The listing builds one solid part. Answer for the finished solid, in the listing's coordinates (mm). A direction names the side the tool comes from. Give positions to 0.01 mm unless a question says otherwise; leave off trailing zeros. Loops run counter-clockwise (first coordinate to the right, second up) from the corner with the lowest first, then second, coordinate; pieces in that order, holes last.
Item 1: Section D-D, the plane x = 0.5 is taken. Give the vertices of the cut face in (y, z), and give its area (3 significant figures).
Item 2: Consider line 1 along X through (y, z) = (-8.25, -46.5); line 2 along Y through (x, z) = (10, -69); line 3 along X through (y, z) = (4.25, -75.5). Determine where each line is inside the solid, lowest interval first.
Item 3: A tool of negligible diameter and unlimited length cuts with its end or side. For faces 5 (the face through (20, -6, -49)), 6 (the face through (13.9, 0, -51)), 7 (the face through (-14, -8.2, -51)), 8 (the face through (-16, -10, -49)), 9 (the face through (10, 3.9, -51)), from which of +Z, -Z, +X, -X, +Y, -Y can it reach the whole face along a straight path? Write none if from no direction.
Item 4: Section C-C, the plane z = -82.5 is taken. Give the number of separate pieces and of enclosed holes in the cut face, and give its area (3 significant figures).
Item 5: Section A-A, the plane x = -10 is taken. Give the vertices of the cut face in (y, z), and give its area (3 significant figures).
Item 6: Section B-B, the plane y = 0 is taken. Give the vertices of the cut face in (x, z), and give its area (3 significant figures).
Item 7: Each of these flat-tipped pins is pushed along its axis until it touches: pin 1 Ø4.5 at (y, z) = (0.5, -52) entering from +X; pin 2 Ø3 at (y, z) = (0.5, -35.5) entering from -X; pin 3 Ø1.2 at (x, z) = (10, -46.5) entering from +Y. Where does it stop, or does it pass through?
Item 8: The mould has two halves that part along Y. Classify faces 1 (the face through (0, -10, -49)), 2 (the face through (-5, 5, 0)), 3 (the face through (-4.49, -4.45, -50.7)), 4 (the face through (5.52, -5.54, -50.7)): pulls with the +Y half, pulls with the -Y half, needs draft (parallel to the pull), parting line crosses it, or undercut.
from build123d import *

# Parameters (mm, degrees)
SKETCH2_W               = 40
SKETCH2_H               = 20
BOSS_EXTRUDE1_DEPTH     = 100
CUT_EXTRUDE1_DEPTH      = 103.46950766
CUT_EXTRUDE1_DEPTH_BACK = 103.46950766
SKETCH3_R               = 2.5
FILLET1_R               = 1.5


with BuildPart() as part:
    # Sketch2 → Boss-Extrude1 (new body)
    with BuildSketch(Plane.XY):
        Rectangle(SKETCH2_W, SKETCH2_H)
    extrude(amount=-BOSS_EXTRUDE1_DEPTH)

    # Sketch3 → Cut-Extrude1 (cut, two sides: drawn at the far end of the back side and taken through both)
    with BuildSketch(Plane.XY.offset(-CUT_EXTRUDE1_DEPTH_BACK)):
        with Locations((-10, 0)):
            Circle(SKETCH3_R)
        with Locations(Location((10, 0, 0), (0, 0, 180))):
            Circle(SKETCH3_R)
        with BuildLine():
            Line((-13.6, 10), (-6.4, 10))
            Line((-6.4, 10), (-6.4, 9.7))
            ThreePointArc((-6.4, 9.7), (-6.458578644, 9.558578644), (-6.6, 9.5))
            Line((-6.6, 9.5), (-6.9, 9.5))
            Line((-6.9, 9.5), (-6.9, 8.2))
            Line((-6.9, 8.2), (-4.5, 8.2))
            Line((-4.5, 8.2), (-4.5, 6.560660172))
            Line((-4.5, 6.560660172), (-6.574873734, 4.485786438))
            ThreePointArc((-6.574873734, 4.485786438), (-7.223720432, 4.052240935), (-7.989087297, 3.9))
            Line((-7.989087297, 3.9), (-12.010912703, 3.9))
            ThreePointArc((-12.010912703, 3.9), (-12.776279568, 4.052240935), (-13.425126266, 4.485786438))
            Line((-13.425126266, 4.485786438), (-15.5, 6.560660172))
            Line((-15.5, 6.560660172), (-15.5, 8.2))
            Line((-15.5, 8.2), (-13.1, 8.2))
            Line((-13.1, 8.2), (-13.1, 9.5))
            Line((-13.1, 9.5), (-13.4, 9.5))
            ThreePointArc((-13.4, 9.5), (-13.541421356, 9.558578644), (-13.6, 9.7))
            Line((-13.6, 9.7), (-13.6, 10))
        make_face()
        with BuildLine():
            Line((-13.6, -10), (-13.6, -9.7))
            ThreePointArc((-13.6, -9.7), (-13.541421356, -9.558578644), (-13.4, -9.5))
            Line((-13.4, -9.5), (-13.1, -9.5))
            Line((-13.1, -9.5), (-13.1, -8.2))
            Line((-13.1, -8.2), (-15.5, -8.2))
            Line((-15.5, -8.2), (-15.5, -6.560660172))
            Line((-15.5, -6.560660172), (-13.425126266, -4.485786438))
            ThreePointArc((-13.425126266, -4.485786438), (-12.776279568, -4.052240935), (-12.010912703, -3.9))
            Line((-12.010912703, -3.9), (-7.989087297, -3.9))
            ThreePointArc((-7.989087297, -3.9), (-7.223720432, -4.052240935), (-6.574873734, -4.485786438))
            Line((-6.574873734, -4.485786438), (-4.5, -6.560660172))
            Line((-4.5, -6.560660172), (-4.5, -8.2))
            Line((-4.5, -8.2), (-6.9, -8.2))
            Line((-6.9, -8.2), (-6.9, -9.5))
            Line((-6.9, -9.5), (-6.6, -9.5))
            ThreePointArc((-6.6, -9.5), (-6.458578644, -9.558578644), (-6.4, -9.7))
            Line((-6.4, -9.7), (-6.4, -10))
            Line((-6.4, -10), (-13.6, -10))
        make_face()
        with BuildLine():
            Line((13.6, -10), (6.4, -10))
            Line((6.4, -10), (6.4, -9.7))
            ThreePointArc((6.4, -9.7), (6.458578644, -9.558578644), (6.6, -9.5))
            Line((6.6, -9.5), (6.9, -9.5))
            Line((6.9, -9.5), (6.9, -8.2))
            Line((6.9, -8.2), (4.5, -8.2))
            Line((4.5, -8.2), (4.5, -6.560660172))
            Line((4.5, -6.560660172), (6.574873734, -4.485786438))
            ThreePointArc((6.574873734, -4.485786438), (7.223720432, -4.052240935), (7.989087297, -3.9))
            Line((7.989087297, -3.9), (12.010912703, -3.9))
            ThreePointArc((12.010912703, -3.9), (12.776279568, -4.052240935), (13.425126266, -4.485786438))
            Line((13.425126266, -4.485786438), (15.5, -6.560660172))
            Line((15.5, -6.560660172), (15.5, -8.2))
            Line((15.5, -8.2), (13.1, -8.2))
            Line((13.1, -8.2), (13.1, -9.5))
            Line((13.1, -9.5), (13.4, -9.5))
            ThreePointArc((13.4, -9.5), (13.541421356, -9.558578644), (13.6, -9.7))
            Line((13.6, -9.7), (13.6, -10))
        make_face()
        with BuildLine():
            Line((13.6, 10), (13.6, 9.7))
            ThreePointArc((13.6, 9.7), (13.541421356, 9.558578644), (13.4, 9.5))
            Line((13.4, 9.5), (13.1, 9.5))
            Line((13.1, 9.5), (13.1, 8.2))
            Line((13.1, 8.2), (15.5, 8.2))
            Line((15.5, 8.2), (15.5, 6.560660172))
            Line((15.5, 6.560660172), (13.425126266, 4.485786438))
            ThreePointArc((13.425126266, 4.485786438), (12.776279568, 4.052240935), (12.010912703, 3.9))
            Line((12.010912703, 3.9), (7.989087297, 3.9))
            ThreePointArc((7.989087297, 3.9), (7.223720432, 4.052240935), (6.574873734, 4.485786438))
            Line((6.574873734, 4.485786438), (4.5, 6.560660172))
            Line((4.5, 6.560660172), (4.5, 8.2))
            Line((4.5, 8.2), (6.9, 8.2))
            Line((6.9, 8.2), (6.9, 9.5))
            Line((6.9, 9.5), (6.6, 9.5))
            ThreePointArc((6.6, 9.5), (6.458578644, 9.558578644), (6.4, 9.7))
            Line((6.4, 9.7), (6.4, 10))
            Line((6.4, 10), (13.6, 10))
        make_face()
        with BuildLine():
            Line((-16.560660172, -5.5), (-18.2, -5.5))
            Line((-18.2, -5.5), (-18.2, -3.1))
            Line((-18.2, -3.1), (-19.5, -3.1))
            Line((-19.5, -3.1), (-19.5, -3.4))
            ThreePointArc((-19.5, -3.4), (-19.558578644, -3.541421356), (-19.7, -3.6))
            Line((-19.7, -3.6), (-20, -3.6))
            Line((-20, -3.6), (-20, 3.6))
            Line((-20, 3.6), (-19.7, 3.6))
            ThreePointArc((-19.7, 3.6), (-19.558578644, 3.541421356), (-19.5, 3.4))
            Line((-19.5, 3.4), (-19.5, 3.1))
            Line((-19.5, 3.1), (-18.2, 3.1))
            Line((-18.2, 3.1), (-18.2, 5.5))
            Line((-18.2, 5.5), (-16.560660172, 5.5))
            Line((-16.560660172, 5.5), (-14.485786438, 3.425126266))
            ThreePointArc((-14.485786438, 3.425126266), (-14.052240935, 2.776279568), (-13.9, 2.010912703))
            Line((-13.9, 2.010912703), (-13.9, -2.010912703))
            ThreePointArc((-13.9, -2.010912703), (-14.052240935, -2.776279568), (-14.485786438, -3.425126266))
            Line((-14.485786438, -3.425126266), (-16.560660172, -5.5))
        make_face()
        with BuildLine():
            Line((14.485786438, -3.425126266), (16.560660172, -5.5))
            Line((16.560660172, -5.5), (18.2, -5.5))
            Line((18.2, -5.5), (18.2, -3.1))
            Line((18.2, -3.1), (19.5, -3.1))
            Line((19.5, -3.1), (19.5, -3.4))
            ThreePointArc((19.5, -3.4), (19.558578644, -3.541421356), (19.7, -3.6))
            Line((19.7, -3.6), (20, -3.6))
            Line((20, -3.6), (20, 3.6))
            Line((20, 3.6), (19.7, 3.6))
            ThreePointArc((19.7, 3.6), (19.558578644, 3.541421356), (19.5, 3.4))
            Line((19.5, 3.4), (19.5, 3.1))
            Line((19.5, 3.1), (18.2, 3.1))
            Line((18.2, 3.1), (18.2, 5.5))
            Line((18.2, 5.5), (16.560660172, 5.5))
            Line((16.560660172, 5.5), (14.485786438, 3.425126266))
            ThreePointArc((14.485786438, 3.425126266), (14.052240935, 2.776279568), (13.9, 2.010912703))
            Line((13.9, 2.010912703), (13.9, -2.010912703))
            ThreePointArc((13.9, -2.010912703), (14.052240935, -2.776279568), (14.485786438, -3.425126266))
        make_face()
        with BuildLine():
            Line((-3.439339828, 8.2), (-3.439339828, 5.5))
            Line((-3.439339828, 5.5), (-5.514213562, 3.425126266))
            ThreePointArc((-5.514213562, 3.425126266), (-5.947759065, 2.776279568), (-6.1, 2.010912703))
            Line((-6.1, 2.010912703), (-6.1, -2.010912703))
            ThreePointArc((-6.1, -2.010912703), (-5.947759065, -2.776279568), (-5.514213562, -3.425126266))
            Line((-5.514213562, -3.425126266), (-3.439339828, -5.5))
            Line((-3.439339828, -5.5), (-3.439339828, -8.2))
            Line((-3.439339828, -8.2), (3.439339828, -8.2))
            Line((3.439339828, -8.2), (3.439339828, -5.5))
            Line((3.439339828, -5.5), (5.514213562, -3.425126266))
            ThreePointArc((5.514213562, -3.425126266), (5.947759065, -2.776279568), (6.1, -2.010912703))
            Line((6.1, -2.010912703), (6.1, 2.010912703))
            ThreePointArc((6.1, 2.010912703), (5.947759065, 2.776279568), (5.514213562, 3.425126266))
            Line((5.514213562, 3.425126266), (3.439339828, 5.5))
            Line((3.439339828, 5.5), (3.439339828, 8.2))
            Line((3.439339828, 8.2), (-3.439339828, 8.2))
        make_face()
    extrude(amount=CUT_EXTRUDE1_DEPTH + CUT_EXTRUDE1_DEPTH_BACK, mode=Mode.SUBTRACT)

    # Fillet1
    fillet1_edges = [part.edges().sort_by_distance(p)[0] for p in [
        (20, -10, -50),
        (-20, -10, -50),
        (-20, 10, -50),
        (20, 10, -50),
    ]]
    fillet(fillet1_edges, radius=FILLET1_R)


solid = part.part
Worked answers:
1. outline: (-10, -100) - (-8.2, -100) - (-8.2, 0) - (-10, 0) - close; (8.2, -100) - (10, -100) - (10, 0) - (8.2, 0) - close
1. area: 360 mm2
2. line 1: x = -20 to -13.1, -6.9 to 6.9, 13.1 to 20
2. line 2: y = -3.9 to -2.5, 2.5 to 3.9
2. line 3: x = -20 to -18.2, -15.31 to -13.14, -6.86 to -4.69, 4.69 to 6.86, 13.14 to 15.31, 18.2 to 20
3. face 5: +Z, -Z, +X, +Y, -Y
3. face 6: +Z, -Z, +X
3. face 7: +Z, -Z
3. face 8: +Z, -Z, +X, -X, -Y
3. face 9: +Z, -Z, +Y
4. separate pieces: 1
4. enclosed holes: 3
4. area: 292 mm2
5. outline: (-3.9, -100) - (-2.5, -100) - (-2.5, 0) - (-3.9, 0) - close; (2.5, -100) - (3.9, -100) - (3.9, 0) - (2.5, 0) - close
5. area: 280 mm2
6. outline: (-13.9, -100) - (-12.5, -100) - (-12.5, 0) - (-13.9, 0) - close; (-7.5, -100) - (-6.1, -100) - (-6.1, 0) - (-7.5, 0) - close; (6.1, -100) - (7.5, -100) - (7.5, 0) - (6.1, 0) - close; (12.5, -100) - (13.9, -100) - (13.9, 0) - (12.5, 0) - close
6. area: 560 mm2
7. pin 1: stops at x = 14.04
7. pin 2: stops at x = -13.9
7. pin 3: stops at y = 3.9
8. face 1: pulls with the -Y half
8. face 2: needs draft
8. face 3: undercut
8. face 4: undercut
